Can you work these out from the model? Positions are in its coordinate system, mm. A direction names the side the tool comes from. Round coordinates to 2 decimals unless told otherwise and drop trailing zeros. Order: outer loops, then holes, each group sorted by start corner. A loop starts at its lowest first (then second) coordinate and runs counter-clockwise, first axis right, second up. Notation, with made-up numbers: M 56.5,50 L 62.5,50 A22 ccw 62.5,61 Z; hole C 67.5,21.5 d10. An arc over 180 degrees is marked long. One line per question, with ' | ' between items.
```python
from build123d import *

# Parameters (mm, degrees)
F0_W     = 762
F0_H     = 2032
F1_DEPTH = 469.9
F2_W     = 419.1
F2_H     = 1117.6
F3_DEPTH = 762
F4_W     = 660.4
F4_H     = 368.3
F5_DEPTH = 2133.6
F6_W     = 660.4
F6_H     = 1117.6
F6_H_2   = 342.9
F6_H_3   = 368.3
F7_DEPTH = 50.801
F8_W     = 660.4
F8_H     = 50.8
F9_DEPTH = 50.8
F11_D    = 5.1054


with BuildPart() as f1:
    # F0 (on Front) → F1 (new body)
    with BuildSketch(Plane.XZ):
        with Locations((381, 1016)):
            Rectangle(F0_W, F0_H)
    extrude(amount=F1_DEPTH)

    # F2 (on face) → F3 (cut)
    with BuildSketch(Plane.YZ.offset(762)):
        with Locations((-260.35, 1422.4)):
            Rectangle(F2_W, F2_H)
        Polygon((-50.8, 50.8), (-50.8, 398.0579510314), (-398.0579510314, 50.8), align=None)
        Polygon((-50.8, 812.8), (-469.9, 812.8), (-469.9, 50.8), (-50.8, 469.9), align=None)
    extrude(amount=-F3_DEPTH, mode=Mode.SUBTRACT)

    # F4 (on face) → F5 (cut)
    with BuildSketch(Plane.XY.offset(2032)):
        with Locations((381, -234.95)):
            Rectangle(F4_W, F4_H)
    extrude(amount=-F5_DEPTH, mode=Mode.SUBTRACT)

    # F6 (on face) → F7 (cut, through all)
    with BuildSketch(Plane.XZ.offset(50.8)):
        with Locations((381, 1422.4)):
            Rectangle(F6_W, F6_H)
        with Locations((381, 641.35)):
            Rectangle(F6_W, F6_H_2)
        with Locations((381, 234.95)):
            Rectangle(F6_W, F6_H_3)
    extrude(amount=-F7_DEPTH, mode=Mode.SUBTRACT)

    # F8 (on face) → F9 (cut)
    with BuildSketch(Plane.XZ.offset(469.9)):
        with Locations((381, 76.2)):
            Rectangle(F8_W, F8_H)
    extrude(amount=-F9_DEPTH, mode=Mode.SUBTRACT)

    # F11 (through all)
    with Locations(Plane(origin=(0, 0, 0), x_dir=(-1, 0, 0), z_dir=(0, 1, 0))):
        with Locations((-397.4977839421, 2003.425), (-364.5022160579, 2003.425), (-92.6977839421, 2003.425), (-29.047275902, 1422.4), (-732.952724098, 1422.4), (-669.3022160579, 841.375), (-397.4977839421, 841.375), (-364.5022160579, 841.375), (-92.6977839421, 841.375), (-669.3022160579, 2003.425)):
            Hole(F11_D / 2)


solid = f1.part
```
(1) If we section it at B-B on z = 1862.5: Please give me the cut outline in (x, y), plus the area to 3 significant figures.
Final values:
outline: M 0,-50.8 L 50.8,-50.8 L 50.8,0 L 0,0 Z; M 711.2,-50.8 L 762,-50.8 L 762,0 L 711.2,0 Z | area: 5,160 mm^2
(2) On a 3-axis mill with a long thin cutter (end or side, diameter ignored), from which of +Z, -Z, +X, -X, +Y, -Y can I reach the whole of each face in a straight line? I mean faces 1 (the flat face through (41, 0, 1096)), 2 (the flat face through (25.8, -263.3, 257.4)), 3 (the flat face through (376, -26, 419.1)), 4 (the flat face through (50.8, -238, 2007)), 5 (the flat face through (0, -147, 861)). Say none if no direction works.
Final values:
face 1: +Z, -Z, +X, -X, +Y | face 2: +X, -X, -Y | face 3: +Y, -Y | face 4: +Z, -Z | face 5: +Z, -Z, -X, +Y, -Y
(3) If we section it at C-C on y = -88: State how many separate pieces and enclosed holes the cut face has, plus the area to 3 significant figures.
Final values:
separate pieces: 8 | enclosed holes: 0 | area: 22,800 mm^2
(4) If we section it at A-A on x = 135: Please give me the cut outline in (y, z).
Final values:
outline: M -469.9,0 L -419.1,0 L -419.1,50.8 L -469.9,50.8 Z; M -469.9,812.8 L -419.1,812.8 L -419.1,863.6 L -469.9,863.6 Z; M -469.9,1981.2 L -419.1,1981.2 L -419.1,2032 L -469.9,2032 Z; M -50.8,0 L 0,0 L 0,50.8 L -50.8,50.8 Z; M -50.8,419.1 L 0,419.1 L 0,469.9 L -50.8,469.9 Z; M -50.8,812.8 L 0,812.8 L 0,863.6 L -50.8,863.6 Z; M -50.8,1981.2 L 0,1981.2 L 0,2032 L -50.8,2032 Z
(5) Please list where these lines run through material, in increasing order: probe 1 along Z at (x, y) = (165, -448); probe 2 along X at (y, z) = (-39, 1302); probe 3 along Y at (x, z) = (685, 824). Write a range as [from, to].
Final values:
probe 1: [0, 50.8], [812.8, 863.6], [1981.2, 2032] | probe 2: [0, 50.8], [711.2, 762] | probe 3: [-469.9, -419.1], [-50.8, 0]
(6) If we section it at D-D on z = 294: Please give me the cut outline in (x, y), plus the area to 3 significant figures.
Final values:
outline: M 0,-226.7 L 50.8,-226.7 L 50.8,-154.86 L 0,-154.86 Z; M 0,-50.8 L 50.8,-50.8 L 50.8,0 L 0,0 Z; M 711.2,-226.7 L 762,-226.7 L 762,-154.86 L 711.2,-154.86 Z; M 711.2,-50.8 L 762,-50.8 L 762,0 L 711.2,0 Z | area: 12,500 mm^2
(7) Thinking about a two-plate mould opening in X: for faces 6 (the flat face through (50.8, -238, 839)), 7 (the flat face through (376, -23, 0)), 8 (the flat face through (762, -147, 861)), which applies, released by +X, released by -X, zero draft, split by the parting line, or undercut?
Final values:
face 6: undercut | face 7: zero draft | face 8: released by +X
